Autodesk Inventor part; units mm, degrees
ref_plane "YZ Plane" through (0, 0, 0) normal (1, 0, 0) x (0, 1, 0)
ref_plane "XZ Plane" through (0, 0, 0) normal (0, 1, 0) x (-1, 0, 0)
ref_plane "XY Plane" through (0, 0, 0) normal (0, 0, 1) x (1, 0, 0)
sketch "Skizze2" plane through (0, 0, 0) normal (0, 1, 0) x (-1, 0, 0)
  line L0 (0, 0) -> (15, 0)
  line L1 (15, 0) -> (15, -5)
  line L2 (15, -5) -> (5, -5)
  line L3 (5, -5) -> (5, -20)
  line L4 (5, -20) -> (0, -20)
  line L5 (0, -20) -> (0, 0)
  dimension "d6" = 5
  dimension "d7" = 15
  dimension "d8" = 5
  dimension "d9" = 10
extrude "Extrusion1" add sketch "Skizze2" along normal blind 112
sketch "Skizze3" plane through (-5, 0, -5) normal (0, 0, -1) x (-1, 0, 0)
  line L0 (0, 112) -> (10, 112)
  line L1 (-5, 0) -> (-5, 112)
  point P0 (5, 99)
  point P1 (5, 70)
  point P2 (5, 41)
  point P3 (5, 12)
  point P4 (5, 112)
  point P5 (5, 112)
  dimension "d12" = 13
  dimension "d13" = 29
  dimension "d14" = 29
  dimension "d15" = 29
  dimension "d39" = 10
hole "Bohrung1" at (-10, 99, -5) at (-10, 70, -5) at (-10, 41, -5) at (-10, 12, -5) direction (0, 0, 1) diameter 4 depth 5 countersink diameter 5 countersink angle 90
sketch "Skizze4" plane through (-5, 0, -20) normal (-1, 0, 0) x (0, 0, 1)
  line L0 (0, 112) -> (15, 112)
  line L1 (0, 0) -> (15, 0)
  line L2 (20, 0) -> (20, 112)
  point P0 (9, 100)
  point P1 (9, 71)
  point P2 (9, 42)
  point P3 (9, 13)
  point P4 (7.5, 0)
  dimension "d30" = 12
  dimension "d31" = 29
  dimension "d32" = 29
  dimension "d33" = 29
  dimension "d40" = 11
hole "Bohrung2" at (-5, 100, -11) at (-5, 71, -11) at (-5, 42, -11) at (-5, 13, -11) direction (1, 0, 0) diameter 5 end through all
fillet "Rundung1" radius 2 2 edges at (-5, 56, -20) (-15, 56, -5)
properties part number "1014"
Here's how the part is built. I have some questions about the finished solid (model axes, mm). Coordinates: 2 decimals unless noted, no trailing zeros. Loops run counter-clockwise (first coordinate to the right, second up) from the corner with the lowest first, then second, coordinate; pieces in that order, holes last. Notation, with made-up numbers: (71.25, -39.5) -> (102.25, -39.5) arc R22 cw to (102.25, -29.5) -> close; hole circle Ø5 at (51.5, -30.75). An arc over 180 degrees is marked (long way). Use one line per item in the form item = value. Start each with the question number.
(1) Please list where these lines run through material, in increasing order: line 1 along Y through (x, z) = (-10, -1.05); line 2 along X through (y, z) = (70, -3.2); line 3 along Z through (x, y) = (-1.05, 100).
(2) If we section it at B-B (x = -1.75): Please give me the cut outline in (y, z).
(3) If we section it at A-A (z = -11): Please give me the cut outline in (x, y).
(4) We'd pull the mould along Y, two halves only. Please class faces 1 (the face through (-4.4, 56.78, -19.43)), 2 (the face through (-2.46, 73.44, -11.54)), 3 (the face through (-4, 0, -8)): pulls with the +Y half, pulls with the -Y half, needs draft (parallel to the pull), parting line crosses it, or undercut.
(5) If we section it at D-D (y = 24): Please give me the cut outline in (x, z).
(6) If we section it at C-C (z = -1.75): Please give me the cut outline in (x, y).
(7) Will these pins go through, and if not, where does the flat tip stop? pin 1 (10.5 mm diameter, centred on y = 36.5, z = -11, fed in from -X); pin 2 (4 mm diameter, centred on x = -10.5, y = 76, fed in from -Z); pin 3 (3 mm diameter, centred on y = 42, z = -11, fed in from -X).
Verdict:
q1.line_1 = 0 to 10, 14 to 39, 43 to 68, 72 to 97, 101 to 112
q1.line_2 = -14.99 to -12, -8 to 0
q1.line_3 = -20 to -13.5, -8.5 to 0
q2.outline = (0, -20) -> (112, -20) -> (112, 0) -> (0, 0) -> close; hole circle Ø5 at (13, -11); hole circle Ø5 at (42, -11); hole circle Ø5 at (71, -11); hole circle Ø5 at (100, -11)
q3.outline = (-5, 0) -> (0, 0) -> (0, 10.5) -> (-5, 10.5) -> close; (-5, 15.5) -> (0, 15.5) -> (0, 39.5) -> (-5, 39.5) -> close; (-5, 44.5) -> (0, 44.5) -> (0, 68.5) -> (-5, 68.5) -> close; (-5, 73.5) -> (0, 73.5) -> (0, 97.5) -> (-5, 97.5) -> close; (-5, 102.5) -> (0, 102.5) -> (0, 112) -> (-5, 112) -> close
q4.face_1 = needs draft
q4.face_2 = undercut
q4.face_3 = pulls with the -Y half
q5.outline = (-15, -3) arc R2 ccw to (-13, -5) -> (-5, -5) -> (-5, -18) arc R2 ccw to (-3, -20) -> (0, -20) -> (0, 0) -> (-15, 0) -> close
q6.outline = (-15, 0) -> (0, 0) -> (0, 112) -> (-15, 112) -> close; hole circle Ø4 at (-10, 12); hole circle Ø4 at (-10, 41); hole circle Ø4 at (-10, 70); hole circle Ø4 at (-10, 99)
q7.pin_1 = -5
q7.pin_2 = -5
q7.pin_3 = through
